Print and shaded views of the part. All mm, measured from the part's lowest x, y and z. A direction names the side the tool comes from. Coordinates: 2 decimals unless noted, no trailing zeros. Order: outer loops, then holes, each group sorted by start corner. A loop starts at its lowest first (then second) coordinate and runs counter-clockwise, first axis right, second up. Notation, with made-up numbers: (18, 31.25) -> (25, 31.25) arc R18 cw to (25, 49.25) -> close; hole circle Ø2 at (-13.75, 17). An arc over 180 degrees is marked (long way). Use one line per item in the form item = value. Start each with the question number.
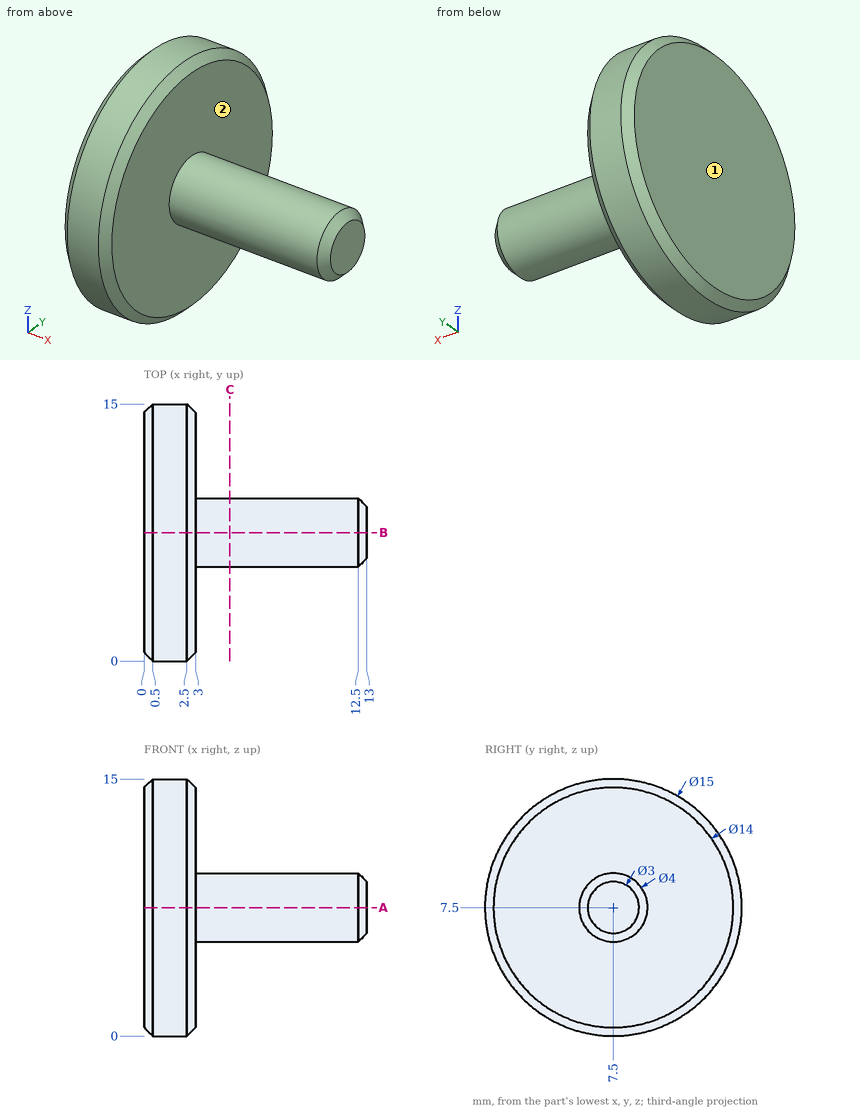
1) Probe L1, parallel to Z at x = 5.5, y = 7.5; L2, parallel to X at y = 11.5, z = 3. List the from-to ranges inside material, lowest first.
2) Cut at C-C on x = 5. Give the cut face in (y, z).
3) Cut at A-A on z = 7.5. Give the cut face in (x, y).
4) Drop flat-ended pins along their axis: P1, Ø4, axis at y = 10, z = 10, coming from the +X side; P2, Ø2, axis at x = 10, y = 6, coming from the +Z side; P3, Ø1, axis at x = 11, y = 9, coming from the +Z side; P4, Ø6, axis at x = 7.5, y = 13, coming from the +Z side. Give the stop position or say it passes through.
5) 3-axis set-ups, long thin cutter, end or side, ignore diameter. For the marked faces 1 and 2: which of +Z, -Z, +X, -X, +Y, -Y reach the whole face in a straight line?
Values follow:
q1.L1 = 5.5 to 9.5
q1.L2 = 0 to 3
q2.outline = circle Ø4 at (7.5, 7.5)
q3.outline = (0, 0.5) -> (0.5, 0) -> (2.5, 0) -> (3, 0.5) -> (3, 5.5) -> (12.5, 5.5) -> (13, 6) -> (13, 9) -> (12.5, 9.5) -> (3, 9.5) -> (3, 14.5) -> (2.5, 15) -> (0.5, 15) -> (0, 14.5) -> close
q4.P1 = 12.96
q4.P2 = 9.44
q4.P3 = 9.23
q4.P4 = through
q5.face_1 = +Z, -Z, -X, +Y, -Y
q5.face_2 = +X
